The model under review builds one solid part; all positions refer to its coordinate system, in mm. Face numbers are marked on the shaded views. A direction names the side the tool comes from. Coordinates: 2 decimals unless noted, no trailing zeros. Order: outer loops, then holes, each group sorted by start corner. A loop starts at its lowest first (then second) coordinate and runs counter-clockwise, first axis right, second up. Notation, with made-up numbers: (-17.5, -31) -> (3.5, -31) arc R27 ccw to (3.5, 3) -> close; hole circle Ø8 at (67, 85). An arc over 180 degrees is marked (long way). Use one line per item in the form item = value. Start each with the question number.
(1) Insertion check: pin 1 Ø1 at (y, z) = (-4, 0) entering from -X; pin 2 Ø2 at (x, z) = (0, 0) entering from +Y; pin 3 Ø1.5 at (y, z) = (-4, 1.5) entering from +X. Each pin has a flat end and moves straight along its axis. Give the tip position at first contact, or say it passes through.
(2) Take a section at A-A (z = 0). State the section outline as (x, y) points.
(3) Take a section at D-D (y = -2). State the section outline as (x, z) points.
(4) Take a section at C-C (y = 1). State the section outline as (x, z) points.
(5) Take a section at B-B (x = 0). State the section outline as (y, z) points, then the cut area to 3 significant figures.
(6) Mouldability with a two-part tool opening along X and no side actions: class the marked faces 3, 4 and 5 as +X half, -X half, draft (parallel to the pull), parting line (faces both ways), or undercut.
(7) Wall thickness on line 1 along X through (y, z) = (7, 0); line 2 along Y through (x, z) = (1.1, 1.3): over which ranges is each line inside the solid? List them lowest first.
(8) For the marked faces 1 and 2, list the 3-axis set-ups (+Z, -Z, +X, -X, +Y, -Y) from which the entire face can be reached by the end or side of a thin tool; tool diameter is ignored.
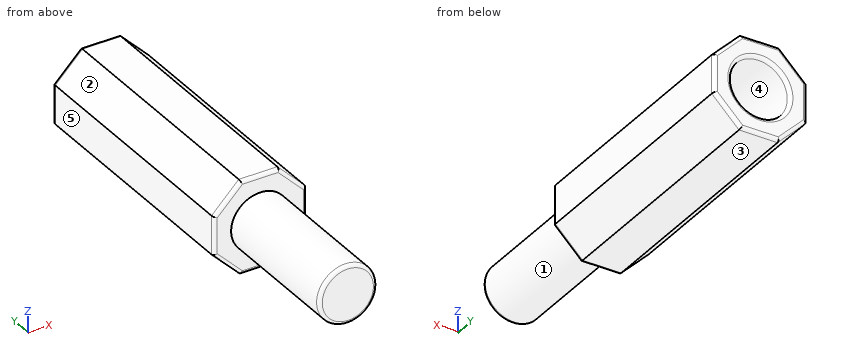
Autodesk Inventor part; units mm, degrees
ref_plane "YZ Plane" through (0, 0, 0) normal (1, 0, 0) x (0, 1, 0)
ref_plane "XZ Plane" through (0, 0, 0) normal (0, 1, 0) x (-1, 0, 0)
ref_plane "XY Plane" through (0, 0, 0) normal (0, 0, 1) x (1, 0, 0)
sketch "Sketch1" plane through (0, 0, 0) normal (0, 1, 0) x (-1, 0, 0)
  line L0 (0.8284, -2) -> (-0.8284, -2)
  line L1 (-0.8284, -2) -> (-2, -0.8284)
  line L2 (-2, -0.8284) -> (-2, 0.8284)
  line L3 (-2, 0.8284) -> (-0.8284, 2)
  line L4 (-0.8284, 2) -> (0.8284, 2)
  line L5 (0.8284, 2) -> (2, 0.8284)
  line L6 (2, 0.8284) -> (2, -0.8284)
  line L7 (2, -0.8284) -> (0.8284, -2)
  point P0 (0, 0)
  point P1 (0, -2)
  point P2 (2, 0)
  dimension "d1" = 135
  dimension "d2" = 4
extrude "Extrusion1" add sketch "Sketch1" along normal blind 11
sketch "Sketch2" plane through (0, 11, 0) normal (0, 1, 0) x (1, 0, 0)
  circle A0 centre (0, 0) radius 1.25
  dimension "d5" = 2.5
extrude "Extrusion2" cut sketch "Sketch2" against normal blind 6.35
thread "Thread1"
sketch "Sketch3" plane through (0, 0, 0) normal (0, -1, 0) x (1, 0, 0)
  circle A0 centre (0, 0) radius 1.25
  dimension "d10" = 2.5
extrude "Extrusion3" add sketch "Sketch3" along normal blind 6
thread "Thread2"
fillet "Fillet1" radius 0.15 16 edges at (1.4142, 11, 1.4142) (2, 11, 0) (1.4142, 11, -1.4142) (0, 11, -2) (-1.4142, 11, -1.4142) (-2, 11, 0) (-1.4142, 11, 1.4142) (0, 11, 2) (1.4142, 0, 1.4142) (0, 0, 2) (-1.4142, 0, 1.4142) (-2, 0, 0) (0, 0, -2) (1.4142, 0, -1.4142) (2, 0, 0) (-1.4142, 0, -1.4142)
fillet "Fillet2" radius 0.15 1 edges at (-1.25, -6, 0)
fillet "Fillet3" radius 0.15 1 edges at (-1.25, 11, 0)
properties part number "11mm M2.5 standoff" material "Steel, High Strength, Low Alloy"
Findings:
q1.pin_1 = -1.25
q1.pin_2 = 4.65
q1.pin_3 = 1
q2.outline = (-2, 0.15) arc R0.15 ccw to (-1.85, 0) -> (-1.25, 0) -> (-1.25, -5.85) arc R0.15 ccw to (-1.1, -6) -> (1.1, -6) arc R0.15 ccw to (1.25, -5.85) -> (1.25, 0) -> (1.85, 0) arc R0.15 ccw to (2, 0.15) -> (2, 10.85) arc R0.15 ccw to (1.85, 11) -> (1.4, 11) arc R0.15 ccw to (1.25, 10.85) -> (1.25, 4.65) -> (-1.25, 4.65) -> (-1.25, 10.85) arc R0.15 ccw to (-1.4, 11) -> (-1.85, 11) arc R0.15 ccw to (-2, 10.85) -> close
q3.outline = circle Ø2.5 at (0, 0)
q4.outline = (-2, -0.83) -> (-0.83, -2) -> (0.83, -2) -> (2, -0.83) -> (2, 0.83) -> (0.83, 2) -> (-0.83, 2) -> (-2, 0.83) -> close
q5.outline = (-6, -1.1) arc R0.15 ccw to (-5.85, -1.25) -> (0, -1.25) -> (0, -1.85) arc R0.15 ccw to (0.15, -2) -> (10.85, -2) arc R0.15 ccw to (11, -1.85) -> (11, -1.4) arc R0.15 ccw to (10.85, -1.25) -> (4.65, -1.25) -> (4.65, 1.25) -> (10.85, 1.25) arc R0.15 ccw to (11, 1.4) -> (11, 1.85) arc R0.15 ccw to (10.85, 2) -> (0.15, 2) arc R0.15 ccw to (0, 1.85) -> (0, 1.25) -> (-5.85, 1.25) arc R0.15 ccw to (-6, 1.1) -> close
q5.area = 43.1 mm²
q6.face_3 = draft
q6.face_4 = undercut
q6.face_5 = -X half
q7.line_1 = -2 to -1.25, 1.25 to 2
q7.line_2 = 0 to 11
q8.face_1 = -Y
q8.face_2 = +Z, -X, +Y, -Y
